Model file for the job. Use its own axes, mm. A direction names the side the tool comes from. Round coordinates to 2 decimals unless told otherwise and drop trailing zeros. Order: outer loops, then holes, each group sorted by start corner. A loop starts at its lowest first (then second) coordinate and runs counter-clockwise, first axis right, second up. Notation, with made-up numbers: M -21.75,61 L 10.25,61 A32 ccw 10.25,96 Z; hole C 51,-10 d8. An arc over 180 degrees is marked long. Return JSON: item names as keys, results as strings. Group by question number.
Item 1: Which spindle directions (+Z, -Z, +X, -X, +Y, -Y) get a long thin tool onto all of the face, cutting with end or side? Do faces 1 (the face through (-171.36, -6.26, 3.13)), 2 (the face through (-147.4, -39.5, 89.034)), 3 (the face through (-138, -71, 6.35)). Say none if no direction does.
Item 2: Slice it at A-A on z = 132.5. Write the cut outline in (x, y) (1 decimal), then the cut area to 3 significant figures.
Item 3: Pin check, flat tips, straight feed: pin 1 Ø7.5 at (x, y) = (-144, -50) entering from +Z; pin 2 Ø7 at (x, y) = (-120, -41) entering from +Z; pin 3 Ø5 at (x, y) = (-148.5, -64.5) entering from -Z. Stop position of each tip, or through.
Item 4: Probe line 1 along Z through (x, y) = (-144, -5); line 2 along Z through (x, y) = (-129, -5); line 3 along Z through (x, y) = (-156.5, -7). List the from-to ranges inside material, lowest first.
Item 5: Slice it at B-B on z = 30. Write the cut outline in (x, y) (1 decimal), then the cut area to 3 significant figures.
Item 6: Pull direction Z, two halves, no side cores. Call faces 4 (the face through (-121, -32, 17.796)), 5 (the face through (-130.467, -34.446, 46.86)), 6 (the face through (-147.2, -38.865, 75.136)): pulls with the +Z half, pulls with the -Z half, needs draft (parallel to the pull), parting line crosses it, or undercut.
from build123d import *

# Parameters (mm, degrees)
F1_ANGLE = 30
F3_DEPTH = 25.4
F5_DEPTH = 25.4


with BuildPart() as f1:
    # F0 (on Front) → F1 (revolve)
    with BuildSketch(Plane.XZ):
        Polygon((-173.0375, 6.35), (-173.0375, 0), (-114.681, 0), (-114.681, 12.7), (-123.5075, 17.795982151), (-128.9685, 17.795982151), (-128.9685, 11.445982151), (-134.9375, 11.445982151), (-134.9375, 81.295982151), (-136.2075, 86.0356866766), (-152.4, 95.3844309105), (-152.4, 89.0344309105), (-157.1625, 89.0344309105), (-157.1625, 158.8844309105), (-173.0375, 158.8844309105), (-173.0375, 152.5344309105), (-163.5125, 143.0094309105), (-163.5125, 86.4041747894), (-141.2875, 64.1791747894), (-141.2875, 6.35), align=None)
    revolve(axis=Axis((0, 0, 96.6527089477), (0, 0, 1)), revolution_arc=F1_ANGLE)

    # F2 (on face) → F3 (cut)
    with BuildSketch(Plane(origin=(0, 0, 0), x_dir=(1, 0, 0), z_dir=(0, 0, -1))):
        with BuildLine():
            Line((-182.2236834316, 21.7005722844), (-168.6606251651, 72.3185948408))
            add(Edge.make_bspline(
                [(-168.6606251651, 72.3185948408), (-206.0052829566, 55.1989492048), (-182.2236834316, 21.7005722844)],
                knots=[0.5949234727, 0.5949234727, 0.5949234727, 2.5466691809, 2.5466691809, 2.5466691809], degree=2, weights=[1, 0.5604453769, 1]))
        make_face()
        with BuildLine():
            add(Edge.make_bspline(
                [(-143.5710023784, 68.2260600336), (-147.7895884166, 72.3535402758), (-153.2578255512, 73.81875)],
                knots=[5.8520567138, 5.8520567138, 5.8520567138, 6.2831853072, 6.2831853072, 6.2831853072], degree=2, weights=[1, 0.9768558474, 1]))
            Line((-153.2578255512, 73.81875), (-143.5710023784, 68.2260600336))
        make_face()
        with BuildLine():
            Line((-158.4491653232, 12.7), (-169.6345452561, 12.7))
            add(Edge.make_bspline(
                [(-169.6345452561, 12.7), (-164.1663081215, 11.2347902758), (-158.4491653232, 12.7)],
                knots=[3.1415926536, 3.1415926536, 3.1415926536, 3.572721247, 3.572721247, 3.572721247], degree=2, weights=[1, 0.9768558474, 1]))
        make_face()
        with BuildLine():
            Line((-143.5710023784, 68.2260600336), (-153.2578255512, 73.81875))
            Line((-153.2578255512, 73.81875), (-169.6345452561, 12.7))
            Line((-169.6345452561, 12.7), (-158.4491653232, 12.7))
            add(Edge.make_bspline(
                [(-158.4491653232, 12.7), (-141.7198075312, 16.987459415), (-136.4732452884, 36.5678954371)],
                knots=[3.572721247, 3.572721247, 3.572721247, 4.7123889674, 4.7123889674, 4.7123889674], degree=2, weights=[1, 0.8419906179, 1]))
            add(Edge.make_bspline(
                [(-136.4732452884, 36.5678954371), (-131.2266828952, 56.1483320204), (-143.5710023784, 68.2260600336)],
                knots=[4.7123889674, 4.7123889674, 4.7123889674, 5.8520567138, 5.8520567138, 5.8520567138], degree=2, weights=[1, 0.8419906109, 1]))
        make_face()
        with BuildLine():
            ThreePointArc((-173.0375, 0), (-172.9018353284, 6.8506748809), (-172.4950540409, 13.6906076446))
            add(Edge.make_bspline(
                [(-182.2236834316, 21.7005722844), (-178.3035736311, 16.1787689453), (-172.4950540409, 13.6906076446)],
                knots=[2.5466691809, 2.5466691809, 2.5466691809, 3.0245373947, 3.0245373947, 3.0245373947], degree=2, weights=[1, 0.9715907886, 1]))
            Line((-182.2236834316, 21.7005722844), (-188.0383342505, 0))
            Line((-188.0383342505, 0), (-173.0375, 0))
        make_face()
        with BuildLine():
            ThreePointArc((-156.2304026489, 74.391113007), (-153.1627191958, 80.5180591843), (-149.8548708073, 86.51875))
            Line((-149.8548708073, 86.51875), (-162.8085898503, 94.1586879635))
            Line((-162.8085898503, 94.1586879635), (-168.6606251651, 72.3185948408))
            add(Edge.make_bspline(
                [(-156.2304026489, 74.391113007), (-162.5048088227, 75.140561907), (-168.6606251651, 72.3185948408)],
                knots=[0.1170552589, 0.1170552589, 0.1170552589, 0.5949234727, 0.5949234727, 0.5949234727], degree=2, weights=[1, 0.9715907886, 1]))
        make_face()
        with BuildLine():
            Line((-153.2578255512, 73.81875), (-149.8548708073, 86.51875))
            ThreePointArc((-149.8548708073, 86.51875), (-153.1627191958, 80.5180591843), (-156.2304026489, 74.391113007))
            add(Edge.make_bspline(
                [(-153.2578255512, 73.81875), (-154.7211037363, 74.210834208), (-156.2304026489, 74.391113007)],
                knots=[0, 0, 0, 0.1170552589, 0.1170552589, 0.1170552589], degree=2, weights=[1, 0.9982877472, 1]))
        make_face()
        with BuildLine():
            Line((-173.0375, 0), (-169.6345452561, 12.7))
            add(Edge.make_bspline(
                [(-172.4950540409, 13.6906076446), (-171.0978234412, 13.092084208), (-169.6345452561, 12.7)],
                knots=[3.0245373947, 3.0245373947, 3.0245373947, 3.1415926536, 3.1415926536, 3.1415926536], degree=2, weights=[1, 0.9982877472, 1]))
            ThreePointArc((-172.4950540409, 13.6906076446), (-172.9018353284, 6.8506748809), (-173.0375, 0))
        make_face()
        with BuildLine():
            Line((-169.6345452561, 12.7), (-153.2578255512, 73.81875))
            add(Edge.make_bspline(
                [(-153.2578255512, 73.81875), (-154.7211037363, 74.210834208), (-156.2304026489, 74.391113007)],
                knots=[0, 0, 0, 0.1170552589, 0.1170552589, 0.1170552589], degree=2, weights=[1, 0.9982877472, 1]))
            ThreePointArc((-156.2304026489, 74.391113007), (-167.1413901665, 44.7854005169), (-172.4950540409, 13.6906076446))
            add(Edge.make_bspline(
                [(-172.4950540409, 13.6906076446), (-171.0978234412, 13.092084208), (-169.6345452561, 12.7)],
                knots=[3.0245373947, 3.0245373947, 3.0245373947, 3.1415926536, 3.1415926536, 3.1415926536], degree=2, weights=[1, 0.9982877472, 1]))
        make_face()
        with BuildLine():
            ThreePointArc((-172.4950540409, 13.6906076446), (-167.1413901665, 44.7854005169), (-156.2304026489, 74.391113007))
            add(Edge.make_bspline(
                [(-156.2304026489, 74.391113007), (-162.5048088227, 75.140561907), (-168.6606251651, 72.3185948408)],
                knots=[0.1170552589, 0.1170552589, 0.1170552589, 0.5949234727, 0.5949234727, 0.5949234727], degree=2, weights=[1, 0.9715907886, 1]))
            Line((-168.6606251651, 72.3185948408), (-182.2236834316, 21.7005722844))
            add(Edge.make_bspline(
                [(-182.2236834316, 21.7005722844), (-178.3035736311, 16.1787689453), (-172.4950540409, 13.6906076446)],
                knots=[2.5466691809, 2.5466691809, 2.5466691809, 3.0245373947, 3.0245373947, 3.0245373947], degree=2, weights=[1, 0.9715907886, 1]))
        make_face()
    extrude(amount=-F3_DEPTH, mode=Mode.SUBTRACT)

    # F4 (on face) → F5 (cut)
    with BuildSketch(Plane.XY.offset(158.8844309105)):
        Polygon((-149.8548708073, -86.51875), (-173.0375, 0), (-187.3384565115, -4.9058394507), (-165.3621643782, -86.51875), align=None)
    extrude(amount=-F5_DEPTH, mode=Mode.SUBTRACT)


solid = f1.part
Output values:
{
 "1": {"face 1": "+Z, -Z, -X, -Y", "face 2": "+Z", "face 3": "-X, -Y"},
 "2": {"outline": "M -163.5,0 A163.5 ccw -141.6,-81.8 L -136.1,-78.6 A157.2 cw -157.2,0 Z", "area": "533 mm²"},
 "3": {"pin 1": "z = 95.38", "pin 2": "z = 17.8", "pin 3": "z = 82.29"},
 "4": {"line 1": "0 to 6.35, 66.98 to 90.58", "line 2": "0 to 11.45", "line 3": "0 to 6.35, 79.55 to 89.03"},
 "5": {"outline": "M -141.3,0 A141.3 ccw -122.4,-70.6 L -116.9,-67.5 A134.9 cw -134.9,0 Z", "area": "459 mm²"},
 "6": {"face 4": "pulls with the +Z half", "face 5": "needs draft", "face 6": "undercut"}
}
